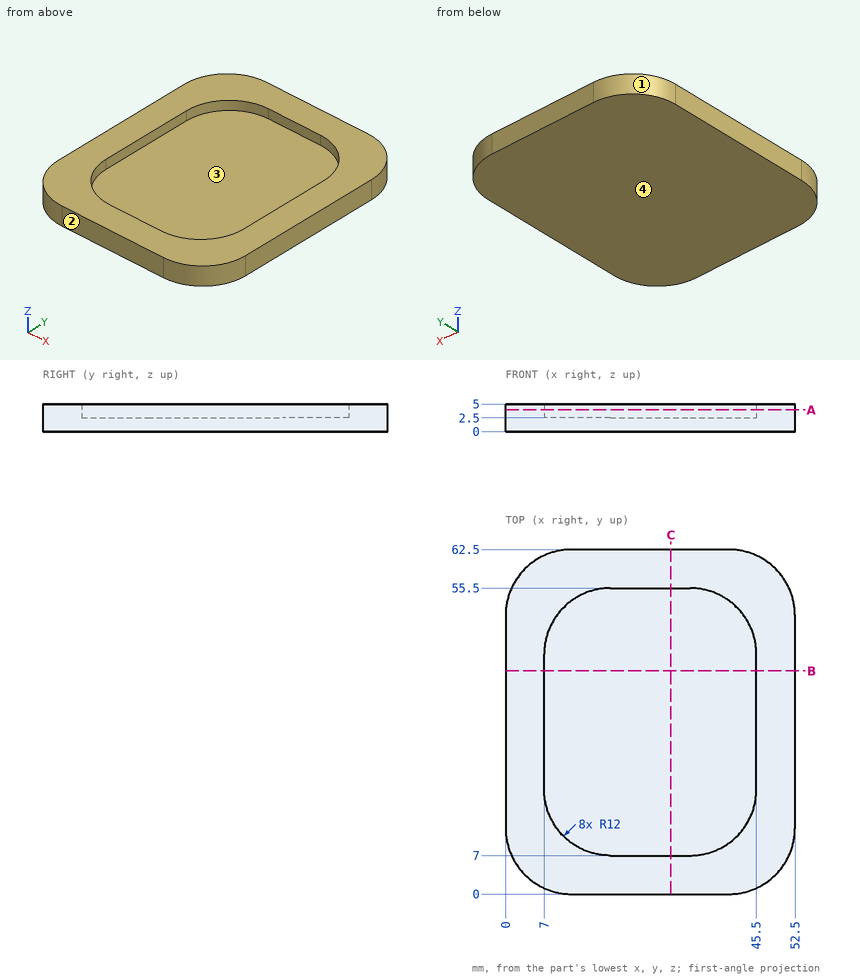
Answer from the drawing. Dimensions are ordinates in mm from the lowest x, y and z of the part. Give positions to 0.01 mm unless a question says otherwise; leave off trailing zeros. Write each loop counter-clockwise with the first axis right and the second up, starting at its lowest first coordinate (ties: lowest second). Pieces come first, ordered by that corner, then holes.
1) For a pull along Y with two mould halves and no side action, classify the marked faces 1, 2, 3 and 4 as pulls with the +Y half, pulls with the -Y half, needs draft (parallel to the pull), parting line crosses it, or undercut.
2) Section A-A (z = 3.95) is taken. Write down the section's boundary in (x, y), and give its area (3 significant figures).
3) Find the intervals of material crossed by L1, parallel to X at y = 41, z = 4.2; L2, parallel to Y at x = 23.5, z = 3; L3, parallel to Z at x = 35.5, y = 16, in increasing order.
4) Given P1, Ø3, axis at x = 25.5, z = 3.5, coming from the -Y side; P2, Ø12, axis at x = 30, y = 14.5, coming from the +Z side, each flat-ended and moving along its own axis, determine where each tip first touches the part or whether it passes through.
5) Section B-B (y = 40.5) is taken. Write down the section's boundary in (x, z), and give its area (3 significant figures).
6) Section C-C (x = 30) is taken. Write down the section's boundary in (y, z), and give its area (3 significant figures).
Response:
1. face 1: pulls with the +Y half
1. face 2: pulls with the -Y half
1. face 3: undercut
1. face 4: needs draft
2. outline: (0, 12) arc R12 ccw to (12, 0) - (40.5, 0) arc R12 ccw to (52.5, 12) - (52.5, 50.5) arc R12 ccw to (40.5, 62.5) - (12, 62.5) arc R12 ccw to (0, 50.5) - close; hole (7, 19) arc R12 ccw to (19, 7) - (33.5, 7) arc R12 ccw to (45.5, 19) - (45.5, 43.5) arc R12 ccw to (33.5, 55.5) - (19, 55.5) arc R12 ccw to (7, 43.5) - close
2. area: 1,410 mm2
3. L1: x = 0 to 7, 45.5 to 52.5
3. L2: y = 0 to 7, 55.5 to 62.5
3. L3: z = 0 to 2.5
4. P1: stops at y = 0
4. P2: stops at z = 2.5
5. outline: (0, 0) - (52.5, 0) - (52.5, 5) - (45.5, 5) - (45.5, 2.5) - (7, 2.5) - (7, 5) - (0, 5) - close
5. area: 166 mm2
6. outline: (0, 0) - (62.5, 0) - (62.5, 5) - (55.5, 5) - (55.5, 2.5) - (7, 2.5) - (7, 5) - (0, 5) - close
6. area: 191 mm2
